Here's how the part is built. I have some questions about the finished solid (model axes, mm). Coordinates: 2 decimals unless noted, no trailing zeros. Loops run counter-clockwise (first coordinate to the right, second up) from the corner with the lowest first, then second, coordinate; pieces in that order, holes last. Notation, with made-up numbers: (60, 85.25) -> (99, 85.25) arc R15 ccw to (99, 91.25) -> close; hole circle Ø7 at (81.25, 10). An arc over 180 degrees is marked (long way). Answer as a JSON object with one key per item and string values. Group by question number.
Q1. I want a section at D-D on z = 8. Write out the boundary of the cut face in (x, y), then the cut area to 3 significant figures.
Q2. I'm going to push a flat-ended pin straight in: pin 1 (9.5 mm diameter, centred on x = 15, z = 37.5, fed in from -Y). Where does the tip first touch, or does it pass through?
Q3. I want a section at B-B on z = -17.5. Write out the boundary of the cut face in (x, y), then the cut area to 3 significant figures.
Q4. I want a section at C-C on x = 0. Write out the boundary of the cut face in (y, z), then the cut area to 3 significant figures.
Q5. I want a section at A-A on y = 1.6. Count the separate pieces of the cut face and the enclosed holes in it, then the cut area to 3 significant figures.
Q6. Thinking about a two-plate mould opening in Z: for faces 1 (the cylindrical face through (-148.57, 2.03, 46)), 2 (the cylindrical face through (-109.513, 1.972, -0.195)), 3 (the flat face through (-64, 0, -1)), which applies, released by +Z, released by -Z, zero draft, split by the parting line, or undercut?
Q7. I need wall thicknesses on line 1 (X direction, y = 3.05, z = -37.5); line 2 (X direction, y = 3, z = 17.5); line 3 (X direction, y = 1.2, z = 4). Which ranges of each line are inside material? Lowest first, please.
```python
from build123d import *

# Parameters (mm, degrees)
SKETCH_1_W      = 175
SKETCH_1_H      = 95
SKETCH_1_R      = 13
SKETCH_1_R_2    = 11
SKETCH_1_R_3    = 2
SKETCH_1_R_4    = 3
SKETCH_1_R_5    = 1.5
EXTRUDE_1_DEPTH = 4
FILLET_1_R      = 5


with BuildPart() as part:
    # 草图1 → 凸台-拉伸1 (new body)
    with BuildSketch(Plane(origin=(0, 0, 0), x_dir=(1, 0, 0), z_dir=(0, 1, 0))):
        with Locations((-62.5, 0)):
            Rectangle(SKETCH_1_W, SKETCH_1_H)
        with Locations(Location((0, 0, 0), (0, 0, 270))):
            Circle(SKETCH_1_R, mode=Mode.SUBTRACT)
        with Locations(Location((-125, 0, 0), (0, 0, 270))):
            Circle(SKETCH_1_R_2, mode=Mode.SUBTRACT)
        with Locations(Location((0, 17.5, 0), (0, 0, 270))):
            Circle(SKETCH_1_R_3, mode=Mode.SUBTRACT)
        with Locations(Location((17.5, 0, 0), (0, 0, 270))):
            Circle(SKETCH_1_R_3, mode=Mode.SUBTRACT)
        with Locations(Location((0, -17.5, 0), (0, 0, 270))):
            Circle(SKETCH_1_R_3, mode=Mode.SUBTRACT)
        with Locations(Location((-17.5, 0, 0), (0, 0, 270))):
            Circle(SKETCH_1_R_3, mode=Mode.SUBTRACT)
        with Locations(Location((-140, 37.5, 0), (0, 0, 270))):
            Circle(SKETCH_1_R_4, mode=Mode.SUBTRACT)
        with Locations(Location((-140, -37.5, 0), (0, 0, 270))):
            Circle(SKETCH_1_R_4, mode=Mode.SUBTRACT)
        with Locations(Location((15, 37.5, 0), (0, 0, 270))):
            Circle(SKETCH_1_R_4, mode=Mode.SUBTRACT)
        with Locations(Location((15, -37.5, 0), (0, 0, 270))):
            Circle(SKETCH_1_R_4, mode=Mode.SUBTRACT)
        with Locations(Location((-125, 14, 0), (0, 0, 270))):
            Circle(SKETCH_1_R_5, mode=Mode.SUBTRACT)
        with Locations(Location((-111, 0, 0), (0, 0, 270))):
            Circle(SKETCH_1_R_5, mode=Mode.SUBTRACT)
        with Locations(Location((-125, -14, 0), (0, 0, 270))):
            Circle(SKETCH_1_R_5, mode=Mode.SUBTRACT)
        with Locations(Location((-139, 0, 0), (0, 0, 270))):
            Circle(SKETCH_1_R_5, mode=Mode.SUBTRACT)
    extrude(amount=EXTRUDE_1_DEPTH)

    # 圆角1
    fillet_1_edges = [part.edges().sort_by_distance(p)[0] for p in [
        (-150, 2, -47.5),
        (25, 2, -47.5),
        (25, 2, 47.5),
        (-150, 2, 47.5),
    ]]
    fillet(fillet_1_edges, radius=FILLET_1_R)


solid = part.part
```
Result set:
{
 "1": {"outline": "(-150, 0) -> (-132.55, 0) -> (-132.55, 4) -> (-150, 4) -> close; (-117.45, 0) -> (-10.25, 0) -> (-10.25, 4) -> (-117.45, 4) -> close; (10.25, 0) -> (25, 0) -> (25, 4) -> (10.25, 4) -> close", "area": "558 mm²"},
 "2": {"pin 1": "stops at y = 0"},
 "3": {"outline": "(-150, 0) -> (-2, 0) -> (-2, 4) -> (-150, 4) -> close; (2, 0) -> (25, 0) -> (25, 4) -> (2, 4) -> close", "area": "684 mm²"},
 "4": {"outline": "(0, -47.5) -> (4, -47.5) -> (4, -19.5) -> (0, -19.5) -> close; (0, -15.5) -> (4, -15.5) -> (4, -13) -> (0, -13) -> close; (0, 13) -> (4, 13) -> (4, 15.5) -> (0, 15.5) -> close; (0, 19.5) -> (4, 19.5) -> (4, 47.5) -> (0, 47.5) -> close", "area": "244 mm²"},
 "5": {"separate pieces": "1", "enclosed holes": "14", "area": "15,500 mm²"},
 "6": {"face 1": "released by +Z", "face 2": "undercut", "face 3": "zero draft"},
 "7": {"line 1": "x = -150 to -143, -137 to 12, 18 to 25", "line 2": "x = -150 to -2, 2 to 25", "line 3": "x = -150 to -135.25, -114.75 to -12.37, 12.37 to 25"}
}
